Read the model definition and answer for the solid it produces. Units are mm, in the model's axes. A direction names the side the tool comes from. Give positions to 0.01 mm unless a question says otherwise; leave off trailing zeros. Order: outer loops, then holes, each group sorted by start corner. A loop starts at its lowest first (then second) coordinate and runs counter-clockwise, first axis right, second up. Notation, with made-up numbers: M 50,55.5 L 79,55.5 A27 ccw 79,83.5 Z; hole C 64.25,28.25 d8. An arc over 180 degrees is marked long. Write item = value, one per line. Start each with the question number.
from build123d import *

# Parameters (mm, degrees)
SKETCH1_R           = 8.89
BOSS_EXTRUDE1_DEPTH = 2.54
BOSS_EXTRUDE2_DEPTH = 5.08


with BuildPart() as part:
    # Sketch1 → Boss-Extrude1 (new body)
    with BuildSketch(Plane(origin=(0, 0, 0), x_dir=(1, 0, 0), z_dir=(0, 1, 0))):
        Circle(SKETCH1_R)
    extrude(amount=BOSS_EXTRUDE1_DEPTH)

    # Sketch2 → Boss-Extrude2 (add)
    with BuildSketch(Plane.XZ):
        with BuildLine():
            Line((-5.470156896, -11.616175324), (1.370506729, -11.61329797))
            Line((1.370506729, -11.61329797), (1.370502542, -11.603343431))
            ThreePointArc((1.370502542, -11.603343431), (10.619701794, -4.872144272), (9.689428275, 6.529229334))
            Line((9.689428275, 6.529229334), (4.409313475, 5.011855517))
            Line((4.409313475, 5.011855517), (2.930122665, 2.816110291))
            ThreePointArc((2.930122665, 2.816110291), (2.540155429, -3.172334534), (-3.388651254, -2.243465774))
            Line((-3.388651254, -2.243465774), (-3.366867699, -2.245362356))
            ThreePointArc((-3.366867699, -2.245362356), (-3.942300227, 0.830594917), (-2.207502202, 3.435035653))
            ThreePointArc((-2.207502202, 3.435035653), (-0.675671449, 5.575210871), (-0.89674169, 8.197801836))
            Line((-0.89674169, 8.197801836), (-3.743562754, 14.29613097))
            ThreePointArc((-3.743562754, 14.29613097), (-7.273662922, 12.829288696), (-10.310746752, 10.507790201))
            ThreePointArc((-10.310746752, 10.507790201), (-14.139706345, 5.222375996), (-15.629256563, -1.131974878))
            ThreePointArc((-15.629256563, -1.131974878), (-12.770870955, -8.526364048), (-5.470156896, -11.616175324))
        make_face()
    extrude(amount=-BOSS_EXTRUDE2_DEPTH)


solid = part.part
1) For a pull along X with two mould halves and no side action, classify faces 4 (the face through (-0.686, 3.792, 5.539)), 5 (the face through (10.55, 2.5, -5.02)), 6 (the face through (7.67, 3.07, 5.95)), 7 (the face through (-2, 0, -1)) as pulls with the +X half, pulls with the -X half, needs draft (parallel to the pull), parting line crosses it, or undercut.
2) Find section B-B on x = -1.5. Determine the outline of the cut face in (y, z).
3) Find the intervals of material crossed by probe 1 along Z at (x, y) = (0, 4); probe 2 along X at (y, z) = (3.15, 0); probe 3 along Y at (x, z) = (3, 5.25), in increasing order. Write a range as [from, to].
4) Find section C-C on z = 0. Determine the outline of the cut face in (x, y).
5) For faces 1 (the face through (-3.95, 3.79, 0.79)), 2 (the face through (3.68, 3.79, 3.93)), 3 (the face through (-14.1, 2.5, 5.31)), determine the directions among +Z, -Z, +X, -X, +Y, -Y from which every point of the face is accessible in a straight line to the end or side of a thin tool.
6) Find section D-D on x = 2.5. Determine the outline of the cut face in (y, z), plus the area to 3 significant figures.
7) Each of these flat-tipped pins is pushed along its axis until it touches: P1, Ø6, axis at x = 0, z = -6, coming from the -Y side; P2, Ø4, axis at x = 3.5, z = 10, coming from the +Y side; P3, Ø1, axis at x = -12.5, y = 0.5, coming from the -Z side. Where does it stop, or does it pass through?
Numbers:
q1.face_4 = undercut
q1.face_5 = pulls with the +X half
q1.face_6 = undercut
q1.face_7 = needs draft
q2.outline = M 0,-11.61 L 5.08,-11.61 L 5.08,-3.78 L 2.54,-3.78 L 2.54,4.06 L 5.08,4.06 L 5.08,9.49 L 0,9.49 Z
q3.probe_1 = [-11.61, -4.06]
q3.probe_2 = [-15.55, -4.03], [4.06, 11.68]
q3.probe_3 = [0, 2.54]
q4.outline = M -15.55,0 L 11.68,0 L 11.68,5.08 L 4.06,5.08 L 4.06,2.54 L -4.03,2.54 L -4.03,5.08 L -15.55,5.08 Z
q5.face_1 = +Y
q5.face_2 = +Z, +Y
q5.face_3 = +Z, -X, +Y, -Y
q6.outline = M 0,-11.41 L 5.08,-11.41 L 5.08,-3.2 L 2.54,-3.2 L 2.54,8.53 L 0,8.53 Z
q6.area = 71.5 mm2
q7.P1 = 0
q7.P2 = 2.54
q7.P3 = -9.24
